Check sheet for the modelled part. Datum: model origin and axes. Units: mm. Face numbers are marked on the shaded views. A direction names the side the tool comes from. Coordinates: 2 decimals unless noted, no trailing zeros. Write each loop counter-clockwise with the first axis right and the second up, starting at its lowest first coordinate (ties: lowest second). Pieces come first, ordered by that corner, then holes. Notation, with made-up numbers: (23.5, 60) -> (82.5, 60) arc R13 ccw to (82.5, 65) -> close; hole circle Ø7 at (9, 47.5). An arc over 180 degrees is marked (long way). One line per item, written item: value. Start each with the question number.
1) Sectioned sample at C-C on x = 35. Enter the section's corners in (y, z), plus the area to 3 significant figures.
2) Sectioned sample at B-B on y = 5.5. Enter the section's corners in (x, z), plus the area to 3 significant figures.
3) Sectioned sample at A-A on z = 33. Enter the section's corners in (x, y), plus the area to 3 significant figures.
4) Set-up check for the marked faces 1 and 2: record each of +Z, -Z, +X, -X, +Y, -Y from which the full face is reachable in a straight line by a thin tool's end or side.
5) Scan lines: line 1 along X through (y, z) = (-6.5, 12.5); line 2 along X through (y, z) = (-1.5, 31.5); line 3 along Z through (x, y) = (-40, 10.5). Record each from-to range of solid material in increasing order. Write a range as [from, to].
6) Gauge pin test, flat ends, axial feed: P1, Ø4, axis at x = -29, z = 21, coming from the +Y side; P2, Ø3, axis at y = -10, z = 42.5, coming from the -X side; P3, Ø2, axis at x = -11.5, y = -23, coming from the +Z side. Record the tip position at first contact, or that the pin passes through.
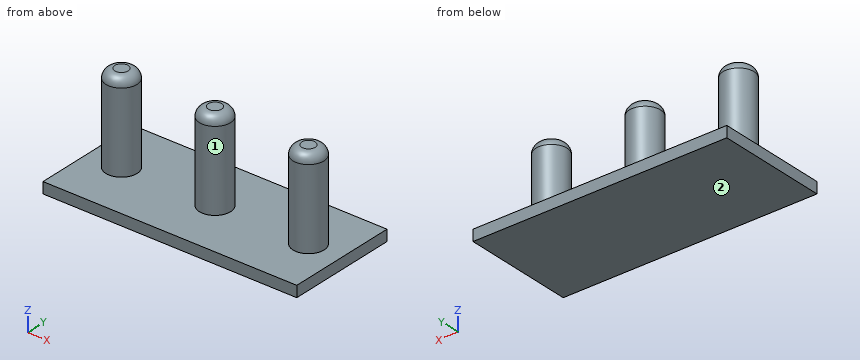
```python
from build123d import *

# Parameters (mm, degrees)
F0_W     = 144.78
F0_H     = 63.5
F1_DEPTH = 6.35
F2_R     = 8.89
F3_DEPTH = 50.8
F4_R     = 5.08


with BuildPart() as f1:
    # F0 (on Top) → F1 (new body)
    with BuildSketch(Plane.XY):
        with Locations((15.891719, -6.567724)):
            Rectangle(F0_W, F0_H)
    extrude(amount=F1_DEPTH)

    # F2 (on face) → F3 (join)
    with BuildSketch(Plane.XY.offset(6.35)):
        with Locations((-37.448281, -6.567724)):
            Circle(F2_R)
        with Locations((15.891719, -6.567724)):
            Circle(F2_R)
        with Locations((69.231719, -6.567724)):
            Circle(F2_R)
    extrude(amount=F3_DEPTH)

    # F4
    f4_edges = [f1.edges().sort_by_distance(p)[0] for p in [
        (60.341719, -6.567724, 57.15),
        (7.001719, -6.567724, 57.15),
        (-46.338281, -6.567724, 57.15),
    ]]
    fillet(f4_edges, radius=F4_R)


solid = f1.part
```
Answers:
1. outline: (-38.32, 0) -> (25.18, 0) -> (25.18, 6.35) -> (-38.32, 6.35) -> close
1. area: 403 mm2
2. outline: (-56.5, 0) -> (88.28, 0) -> (88.28, 6.35) -> (-56.5, 6.35) -> close
2. area: 919 mm2
3. outline: circle Ø17.78 at (-37.45, -6.57); circle Ø17.78 at (15.89, -6.57); circle Ø17.78 at (69.23, -6.57)
3. area: 745 mm2
4. face 1: +Z
4. face 2: -Z, +X, -X, +Y, -Y
5. line 1: x = [-46.34, -28.56], [7, 24.78], [60.34, 78.12]
5. line 2: x = [-44.75, -30.14], [8.59, 23.2], [61.93, 76.54]
5. line 3: z = [0, 6.35]
6. P1: stops at y = -0.45
6. P2: stops at x = -46.13
6. P3: stops at z = 6.35
